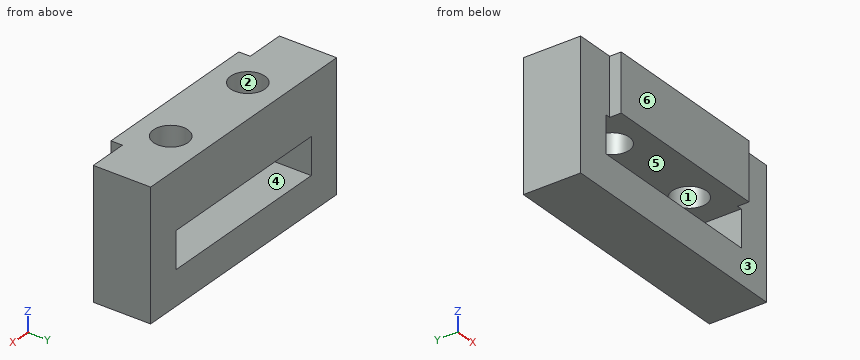
```python
from build123d import *

# Parameters (mm, degrees)
SKETCH_1_W      = 15.12
SKETCH_1_H      = 6
SKETCH_1_R      = 1.5
EXTRUDE_1_DEPTH = 5
EXTRUDE_2_DEPTH = 5


with BuildPart() as part:
    # Эскиз1 → Бобышка-Вытянуть1 (new body)
    with BuildSketch(Plane.XY):
        with Locations((4.56, 0)):
            Rectangle(SKETCH_1_W, SKETCH_1_H)
        Circle(SKETCH_1_R, mode=Mode.SUBTRACT)
        with Locations((9.12, 0)):
            Circle(SKETCH_1_R, mode=Mode.SUBTRACT)
    extrude(amount=EXTRUDE_1_DEPTH)

    # Эскиз2 → Бобышка-Вытянуть2 (add)
    with BuildSketch(Plane(origin=(0, 3, 0), x_dir=(1, 0, 0), z_dir=(0, 1, 0))):
        Polygon((12.12, -5), (15.56, -5), (15.56, 6.2), (-6.44, 6.2), (-6.44, -5), (-3, -5), (-3, 0), (-3.44, 0), (-3.44, 3.2), (12.56, 3.2), (12.56, 0), (12.12, 0), align=None)
    extrude(amount=-EXTRUDE_2_DEPTH)


solid = part.part
```
The model under review builds one solid part; all positions refer to its coordinate system, in mm. Face numbers are marked on the shaded views. A direction names the side the tool comes from. Give positions to 0.01 mm unless a question says otherwise; leave off trailing zeros. Write each loop counter-clockwise with the first axis right and the second up, starting at its lowest first coordinate (ties: lowest second). Pieces come first, ordered by that corner, then holes. Notation, with made-up numbers: (78, 45.5) - (106, 45.5) arc R33 ccw to (106, 80.5) - close; hole circle Ø9 at (-37.75, 45.25). An arc over 180 degrees is marked (long way). Answer in a Markdown table with one row per item. Add a question column.
1. We need section C-C on x = 5.5. Write out the cut boundary in (y, z).
2. Tool access review of the marked faces 5 and 6: name each direction out of +Z, -Z, +X, -X, +Y, -Y from which nothing blocks a thin tool from reaching the whole face with its end or side.
3. We need section D-D on y = 2.2. Write out the cut boundary in (x, z), then the cut area to 3 significant figures.
4. We need section A-A on y = 0. Write out the cut boundary in (x, z), then the cut area to 3 significant figures.
5. We need section B-B on z = -0.75. Write out the cut boundary in (x, y).
6. Wall thickness on line 1 along X through (y, z) = (0.1, 4.5); line 2 along Z through (x, y) = (4, -0.5); line 3 along Y through (x, z) = (0, 3.9): over which ranges is each line inside the solid? List them lowest first. Write a range as [from, to].
7. Draft analysis for pull direction Y (two halves, no side actions). For the marked faces 1, 2, 3 and 4, state which applies: +Y half, -Y half, draft (parallel to the pull), parting line (faces both ways), or undercut.
8. Insertion check: P1, Ø0.8, axis at y = -2.5, z = 2, coming from the -X side; P2, Ø0.8, axis at y = -2.5, z = 2, coming from the +X side. Each pin has a flat end and moves straight along its axis. Give the tip position at first contact, or say it passes through.
Ans:
| question | item | result |
|---|---|---|
| 1 | outline | (-3, 0) - (3, 0) - (3, 5) - (-3, 5) - close; (-2, -6.2) - (3, -6.2) - (3, -3.2) - (-2, -3.2) - close |
| 2 | face 5 | +Y, -Y |
| 2 | face 6 | +Z, -Z, +X, -X, -Y |
| 3 | outline | (-6.44, -6.2) - (15.56, -6.2) - (15.56, 5) - (-6.44, 5) - close; hole (-3.44, -3.2) - (12.56, -3.2) - (12.56, 0) - (-3.44, 0) - close |
| 3 | area | 195 mm^2 |
| 4 | outline | (-6.44, -6.2) - (15.56, -6.2) - (15.56, 5) - (10.62, 5) - (10.62, 0) - (12.56, 0) - (12.56, -3.2) - (-3.44, -3.2) - (-3.44, 0) - (-1.5, 0) - (-1.5, 5) - (-6.44, 5) - close; (1.5, 0) - (7.62, 0) - (7.62, 5) - (1.5, 5) - close |
| 4 | area | 165 mm^2 |
| 5 | outline | (-6.44, -2) - (-3.44, -2) - (-3.44, 3) - (-6.44, 3) - close; (12.56, -2) - (15.56, -2) - (15.56, 3) - (12.56, 3) - close |
| 6 | line 1 | x = [-6.44, -1.5], [1.5, 7.62], [10.62, 15.56] |
| 6 | line 2 | z = [-6.2, -3.2], [0, 5] |
| 6 | line 3 | y = [-3, -1.5], [1.5, 3] |
| 7 | face 1 | undercut |
| 7 | face 2 | undercut |
| 7 | face 3 | -Y half |
| 7 | face 4 | draft |
| 8 | P1 | stops at x = -3 |
| 8 | P2 | stops at x = 12.12 |
